Geometry check sheet. Reference: the model listing, model coordinates, mm. A direction names the side the tool comes from. Give positions to 0.01 mm unless a question says otherwise; leave off trailing zeros. Loops run counter-clockwise (first coordinate to the right, second up) from the corner with the lowest first, then second, coordinate; pieces in that order, holes last. Notation, with made-up numbers: (86, 15) - (97, 15) arc R31 cw to (97, 49) - close; hole circle Ø4 at (50.5, 85.5). An arc over 180 degrees is marked (long way). Use a Markdown table: item, result. Add a question column.
1. Material ranges on L1, parallel to Z at x = 32, y = 1.15; L2, parallel to X at y = 1.6, z = 16; L3, parallel to X at y = 18.5, z = 30, recorded low to high.
2. Depth check by flat-ended pin: P1, Ø2.5, axis at x = -32, z = 16, coming from the +Y side; P2, Ø6, axis at x = -21.5, z = 3.5, coming from the -Y side; P3, Ø6, axis at y = 11.5, z = 3, coming from the -X side; P4, Ø1.5, axis at y = 14, z = -6, coming from the +X side. Enter the tip coordinate at first touch or a pass-through.
3. Set-up check for faces 4 (the flat face through (-30, 3, 1)), 5 (the flat face through (26, 13, 1)), 6 (the flat face through (-36, 1, -1)): record each of +Z, -Z, +X, -X, +Y, -Y from which the full face is reachable in a straight line by a thin tool's end or side.
4. Draft check along Z on faces 1 (the cylindrical face through (34, 2, 16)), 2 (the flat face through (-1, 11, 36)), 3 (the flat face through (-26, 13, -1)). Enter one of: pulls with the +Z half, pulls with the -Z half, needs draft (parallel to the pull), parting line crosses it, or undercut.
5. Cross-section at B-B on x = -32. Enter the section's corners in (y, z), and give its area (3 significant figures).
6. Cross-section at A-A on z = 32. Enter the section's corners in (x, y), and give its area (3 significant figures).
7. Cross-section at C-C on y = 2. Count the separate pieces of the cut face and the enclosed holes in it, and give its area (3 significant figures).
8. Cross-section at D-D on z = -21.5. Enter the section's corners in (x, y).
Autodesk Inventor part; units mm, degrees
ref_plane "YZ Plane" through (0, 0, 0) normal (1, 0, 0) x (0, 1, 0)
ref_plane "XZ Plane" through (0, 0, 0) normal (0, 1, 0) x (-1, 0, 0)
ref_plane "XY Plane" through (0, 0, 0) normal (0, 0, 1) x (1, 0, 0)
sketch "Sketch1" plane through (0, 0, 0) normal (0, 1, 0) x (-1, 0, 0)
  line L0 (-36, -36) -> (36, -36)
  line L1 (36, -36) -> (36, 36)
  line L2 (36, 36) -> (-36, 36)
  line L3 (-36, 36) -> (-36, -36)
  line L4 (-36, -36) -> (36, 36) construction
  line L5 (36, -36) -> (-36, 36) construction
  point P0 (0, 0)
  dimension "d0" = 72
  dimension "d1" = 72
extrude "Extrusion1" add sketch "Sketch1" along normal blind 3
sketch "Sketch2" plane through (0, 3, 0) normal (0, 1, 0) x (1, 0, 0)
  line L0 (-36, -36) -> (36, -36)
  line L1 (26, 36) -> (-26, 36)
  line L2 (-26, 36) -> (-26, -36)
  line L3 (-26, -36) -> (26, -36)
  line L4 (26, -36) -> (26, 36)
  line L5 (26, 36) -> (-26, -36) construction
  line L6 (-26, 36) -> (26, -36) construction
  point P0 (0, 0)
  dimension "d4" = 52
extrude "Extrusion2" add sketch "Sketch2" along normal blind 20
sketch "Sketch3" plane through (0, 0, 0) normal (0, -1, 0) x (1, 0, 0)
  line L0 (-36, 36) -> (36, 36)
  line L1 (-36, 36) -> (-32, 36)
  line L2 (-32, 36) -> (-32, 32)
  line L3 (-32, 32) -> (-36, 32)
  line L4 (-36, 32) -> (-36, 36)
  circle A0 centre (-32, 16) radius 1.85
  circle A1 centre (-32, 0) radius 1.85
  circle A2 centre (-32, -16) radius 1.85
  circle A3 centre (-32, -32) radius 1.85
  point P0 (0, 0)
  dimension "d7" = 4
  dimension "d8" = 4
hole "Hole2" at (-32, 0, 32) at (-32, 0, 16) at (-32, 0, 0) at (-32, 0, -16) at (-32, 0, -32) direction (0, 1, 0) diameter 4 end through all
sketch "Sketch4" plane through (0, 0, 0) normal (0, -1, 0) x (1, 0, 0)
  circle A0 centre (32, -32) radius 1.85
  circle A1 centre (32, -16) radius 1.85
  circle A2 centre (32, 0) radius 1.85
  circle A3 centre (32, 16) radius 1.85
  circle A4 centre (32, 32) radius 1.85
  point P0 (0, 0)
hole "Hole4" at (32, 0, 32) at (32, 0, 16) at (32, 0, 0) at (32, 0, -16) at (32, 0, -32) direction (0, 1, 0) diameter 4 end through all
properties part number "Legacy Module"
Values found:
| question | item | result |
|---|---|---|
| 1 | L1 | z = -36 to -34, -30 to -18, -14 to -2, 2 to 14, 18 to 30, 34 to 36 |
| 1 | L2 | x = -36 to -34, -30 to 30, 34 to 36 |
| 1 | L3 | x = -26 to 26 |
| 2 | P1 | passes through |
| 2 | P2 | stops at y = 0 |
| 2 | P3 | stops at x = -26 |
| 2 | P4 | stops at x = 26 |
| 3 | face 4 | +Z, -Z, -X, +Y |
| 3 | face 5 | +Z, -Z, +X, +Y |
| 3 | face 6 | +Z, -Z, -X, +Y, -Y |
| 4 | face 1 | undercut |
| 4 | face 2 | pulls with the +Z half |
| 4 | face 3 | needs draft |
| 5 | outline | (0, -36) - (3, -36) - (3, -34) - (0, -34) - close; (0, -30) - (3, -30) - (3, -18) - (0, -18) - close; (0, -14) - (3, -14) - (3, -2) - (0, -2) - close; (0, 2) - (3, 2) - (3, 14) - (0, 14) - close; (0, 18) - (3, 18) - (3, 30) - (0, 30) - close; (0, 34) - (3, 34) - (3, 36) - (0, 36) - close |
| 5 | area | 156 mm2 |
| 6 | outline | (-36, 0) - (-34, 0) - (-34, 3) - (-36, 3) - close; (-30, 0) - (30, 0) - (30, 3) - (26, 3) - (26, 23) - (-26, 23) - (-26, 3) - (-30, 3) - close; (34, 0) - (36, 0) - (36, 3) - (34, 3) - close |
| 6 | area | 1,230 mm2 |
| 7 | separate pieces | 1 |
| 7 | enclosed holes | 10 |
| 7 | area | 5,060 mm2 |
| 8 | outline | (-36, 0) - (36, 0) - (36, 3) - (26, 3) - (26, 23) - (-26, 23) - (-26, 3) - (-36, 3) - close |
